```python
from build123d import *

# Parameters (mm, degrees)
F1_DEPTH = 4.318
F2_R     = 3.175
F2_R_2   = 1.1303
F3_DEPTH = 6.35
F4_R     = 2.1971
F5_DEPTH = 1.27
F6_R     = 1.1303
F7_DEPTH = 25.4


with BuildPart() as f1:
    # F0 (on Front) → F1 (new body)
    with BuildSketch(Plane.XZ):
        Polygon((3.299557, 5.715), (-3.299557, 5.715), (-6.599114, 0), (-3.299557, -5.715), (3.299557, -5.715), (6.599114, 0), align=None)
    extrude(amount=F1_DEPTH)

    # F2 (on face) → F3 (join)
    with BuildSketch(Plane.XZ.offset(4.318)):
        Circle(F2_R)
        Circle(F2_R_2, mode=Mode.SUBTRACT)
    extrude(amount=F3_DEPTH)

    # F4 (on face) → F5 (cut)
    with BuildSketch(Plane(origin=(0, 0, 0), x_dir=(-1, 0, 0), z_dir=(0, 1, 0))):
        Circle(F4_R)
    extrude(amount=-F5_DEPTH, mode=Mode.SUBTRACT)

    # F6 (on face) → F7 (cut)
    with BuildSketch(Plane(origin=(0, -1.27, 0), x_dir=(-1, 0, 0), z_dir=(0, 1, 0))):
        Circle(F6_R)
    extrude(amount=-F7_DEPTH, mode=Mode.SUBTRACT)


solid = f1.part
```
Work out the finished part from the listing and answer in its coordinate system (mm). A direction names the side the tool comes from. Round coordinates to 2 decimals unless told otherwise and drop trailing zeros. Write each loop counter-clockwise with the first axis right and the second up, starting at its lowest first coordinate (ties: lowest second). Pieces come first, ordered by that corner, then holes. Notation, with made-up numbers: (12, 39) - (23, 39) arc R9 ccw to (23, 52) - close; hole circle Ø7 at (62.25, -28.75). An arc over 180 degrees is marked (long way). Return JSON: item names as keys, results as strings. Group by question number.
Q1. For faces 5 (the cylindrical face through (-0.69, -7.45, -3.1)), 6 (the flat face through (1, -1.27, 1)), 7 (the flat face through (-4.926, -2.129, 2.898)), determine the directions among +Z, -Z, +X, -X, +Y, -Y from which every point of the face is accessible in a straight line to the end or side of a thin tool.
Q2. The part is cut by section B-B on x = 0. Write down the section's boundary in (y, z) (3 decimals), then the cut area to 3 significant figures.
Q3. Find the intervals of material crossed by L1, parallel to Z at x = 0, y = -5.25 (3 decimals); L2, parallel to Z at x = 0, y = -0.8 (3 decimals); L3, parallel to Y at x = 1, z = -1.5, in increasing order.
Q4. The part is cut by section C-C on z = 0.25. Write down the section's boundary in (x, y).
Q5. The mould has two halves that part along Z. Classify faces 1 (the flat face through (0, -2, 5.715)), 2 (the flat face through (3, 0, 0)), 3 (the cylindrical face through (0.476, -0.626, -2.145)), 4 (the cylindrical face through (0.245, -5.903, -1.103)): released by +Z, released by -Z, zero draft, split by the parting line, or undercut.
Q6. The part is cut by section A-A on y = -1. Write down the section's boundary in (x, z) (3 decimals), then the cut area to 3 significant figures.
Q7. The part is cut by section D-D on y = -3.25. Write down the section's boundary in (x, z) (3 decimals), then the cut area to 3 significant figures.
Q8. This flat-tipped pin is pushed along its axis until it touches: pin 1 Ø5 at (x, z) = (0, 0) entering from -Y. Where does it stop, or does it pass through?
Solved:
{
 "1": {"face 5": "-Y", "face 6": "+Y", "face 7": "+Z, -X, +Y, -Y"},
 "2": {"outline": "(-10.668, -3.175) - (-4.318, -3.175) - (-4.318, -5.715) - (0, -5.715) - (0, -2.197) - (-1.27, -2.197) - (-1.27, -1.13) - (-10.668, -1.13) - close; (-10.668, 1.13) - (-1.27, 1.13) - (-1.27, 2.197) - (0, 2.197) - (0, 5.715) - (-4.318, 5.715) - (-4.318, 3.175) - (-10.668, 3.175) - close", "area": "62.9 mm²"},
 "3": {"L1": "-3.175 to -1.13, 1.13 to 3.175", "L2": "-5.715 to -2.197, 2.197 to 5.715", "L3": "-10.67 to -1.27"},
 "4": {"outline": "(-6.45, -4.32) - (-3.17, -4.32) - (-3.17, -10.67) - (-1.1, -10.67) - (-1.1, -1.27) - (-2.18, -1.27) - (-2.18, 0) - (-6.45, 0) - close; (1.1, -10.67) - (3.17, -10.67) - (3.17, -4.32) - (6.45, -4.32) - (6.45, 0) - (2.18, 0) - (2.18, -1.27) - (1.1, -1.27) - close"},
 "5": {"face 1": "released by +Z", "face 2": "zero draft", "face 3": "undercut", "face 4": "undercut"},
 "6": {"outline": "(-6.599, 0) - (-3.3, -5.715) - (3.3, -5.715) - (6.599, 0) - (3.3, 5.715) - (-3.3, 5.715) - close; hole circle Ø4.394 at (0, 0)", "area": "98.0 mm²"},
 "7": {"outline": "(-6.599, 0) - (-3.3, -5.715) - (3.3, -5.715) - (6.599, 0) - (3.3, 5.715) - (-3.3, 5.715) - close; hole circle Ø2.261 at (0, 0)", "area": "109 mm²"},
 "8": {"pin 1": "y = -10.67"}
}
